The figure shows three views and two pictorial views of one solid part (mm, origin at its lowest corner). Answer the questions. A direction names the side the tool comes from. Coordinates: 2 decimals unless noted, no trailing zeros. Order: outer loops, then holes, each group sorted by start corner. A loop starts at its lowest first (then second) coordinate and runs counter-clockwise, first axis right, second up.
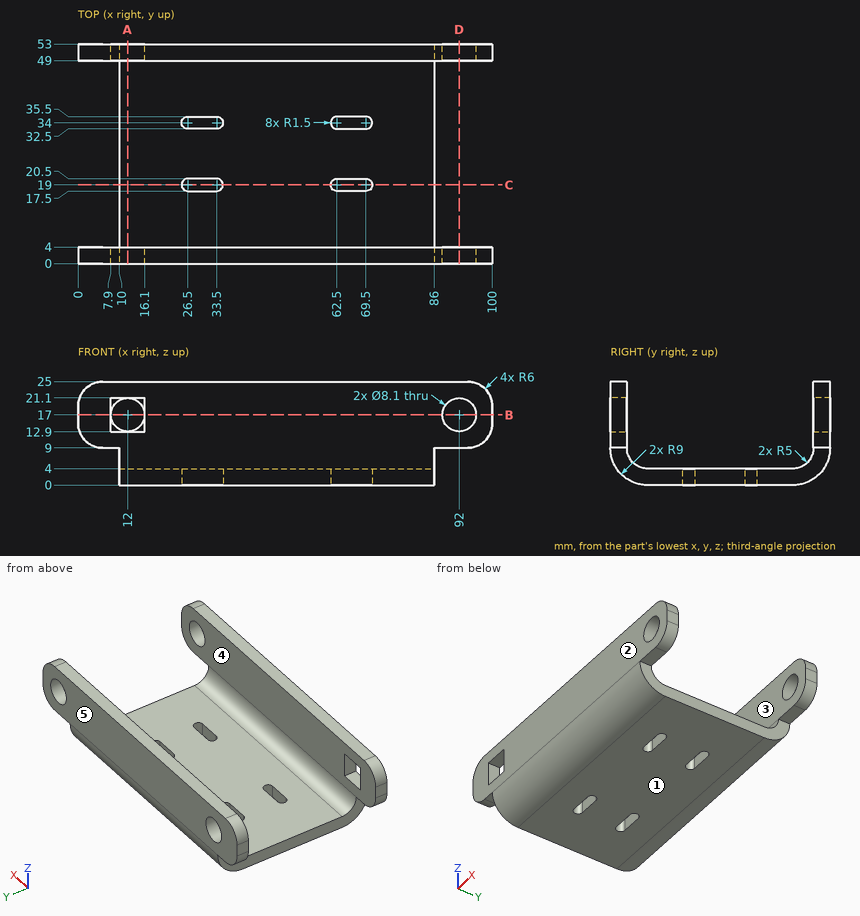
Q1. Which of the six approach directions +Z, -Z, +X, -X, +Y, -Y give full straight-line access (tool end or side, diameter ignored) to the marked faces 4 and 5?
Q2. The part is cut by section B-B, the plane z = 17. Determine the outline of the cut face in (x, y), then the cut area to 3 significant figures.
Q3. The part is cut by section D-D, the plane x = 92. Determine the outline of the cut face in (y, z).
Q4. Straight lines are drawn through the part: L1, parallel to X at y = 51.45, z = 17; L2, parallel to X at y = 1.6, z = 17; L3, parallel to Y at x = 93.5, z = 10.75. For each, find the intervals that lie inside material, in ascending order.
Q5. The part is cut by section A-A, the plane x = 12. Determine the outline of the cut face in (y, z).
Q6. Determine the mould class of the marked faces 1, 2 and 3 for opening direction Y: +Y half, -Y half, draft (parallel to the pull), parting line (faces both ways), or undercut.
Q7. Each of these flat-tipped pins is pushed along its axis until it touches: P1, Ø6, axis at x = 61, z = 4.5, coming from the -Y side; P2, Ø1.2, axis at x = 13.5, y = 2.5, coming from the -Z side; P3, Ø4.5, axis at x = 66.5, z = 1, coming from the -Y side; P4, Ø7.5, axis at x = 92, z = 17, coming from the -Y side. Where does it stop, or does it pass through?
Q8. The part is cut by section C-C, the plane y = 19. Determine the outline of the cut face in (x, z).
Computed values:
1. face 4: +Z, +X, -X
1. face 5: +Z, -Z, +X, -X, +Y
2. outline: (0, 0) - (7.9, 0) - (7.9, 4) - (0, 4) - close; (0, 49) - (7.95, 49) - (7.95, 53) - (0, 53) - close; (16.05, 49) - (87.95, 49) - (87.95, 53) - (16.05, 53) - close; (16.1, 0) - (87.95, 0) - (87.95, 4) - (16.1, 4) - close; (96.05, 0) - (100, 0) - (100, 4) - (96.05, 4) - close; (96.05, 49) - (100, 49) - (100, 53) - (96.05, 53) - close
2. area: 670 mm2
3. outline: (0, 9) - (4, 9) - (4, 12.95) - (0, 12.95) - close; (0, 21.05) - (4, 21.05) - (4, 25) - (0, 25) - close; (49, 9) - (53, 9) - (53, 12.95) - (49, 12.95) - close; (49, 21.05) - (53, 21.05) - (53, 25) - (49, 25) - close
4. L1: x = 0 to 7.95, 16.05 to 87.95, 96.05 to 100
4. L2: x = 0 to 7.9, 16.1 to 87.95, 96.05 to 100
4. L3: y = 0 to 4, 49 to 53
5. outline: (0, 9) arc R9 ccw to (9, 0) - (44, 0) arc R9 ccw to (53, 9) - (53, 12.95) - (49, 12.95) - (49, 9) arc R5 cw to (44, 4) - (9, 4) arc R5 cw to (4, 9) - (4, 12.9) - (0, 12.9) - close; (0, 21.1) - (4, 21.1) - (4, 25) - (0, 25) - close; (49, 21.05) - (53, 21.05) - (53, 25) - (49, 25) - close
6. face 1: draft
6. face 2: -Y half
6. face 3: undercut
7. P1: stops at y = 0.13
7. P2: stops at z = 2.2
7. P3: stops at y = 2.08
7. P4: passes through
8. outline: (10, 0) - (25, 0) - (25, 4) - (10, 4) - close; (35, 0) - (61, 0) - (61, 4) - (35, 4) - close; (71, 0) - (86, 0) - (86, 4) - (71, 4) - close
